Read the model definition and answer for the solid it produces. Units are mm, in the model's axes. Face numbers are marked on the shaded views. Coordinates: 2 decimals unless noted, no trailing zeros. Order: outer loops, then holes, each group sorted by start corner. A loop starts at its lowest first (then second) coordinate and runs counter-clockwise, first axis right, second up. Notation, with made-up numbers: (16, -32.5) -> (44, -32.5) arc R20 cw to (44, 0.5) -> close; hole circle Ø3 at (45.25, -31.75). An arc over 180 degrees is marked (long way). Use CSV: the item, a comma, the result in double quotes.
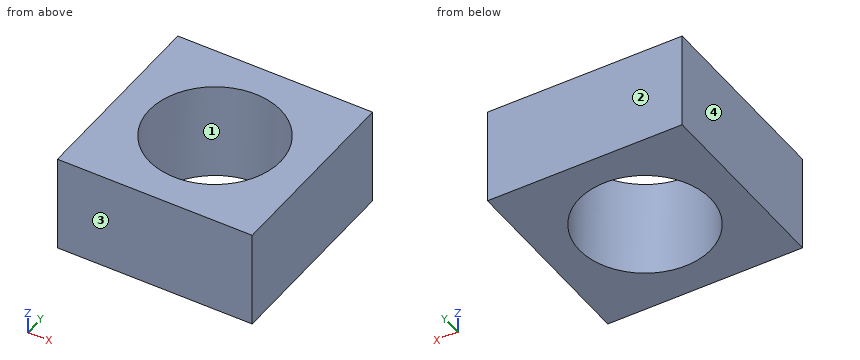
```python
from build123d import *

# Parameters (mm, degrees)
SKETCH2_W                       = 8
SKETCH2_H                       = 8
REFERENCE_SQUARE_NUT_DEPTH      = 4
SKETCH3_R                       = 2.7
SIMPLIFIED_CLEARANCE_BORE_DEPTH = 4


with BuildPart() as part:
    # Sketch2 → Reference_square_nut (new body)
    with BuildSketch(Plane.XY):
        Rectangle(SKETCH2_W, SKETCH2_H)
    extrude(amount=REFERENCE_SQUARE_NUT_DEPTH)

    # Sketch3 → Simplified_clearance_bore (cut)
    with BuildSketch(Plane.XY):
        Circle(SKETCH3_R)
    extrude(amount=SIMPLIFIED_CLEARANCE_BORE_DEPTH, mode=Mode.SUBTRACT)


solid = part.part
```
Item 1: Straight lines are drawn through the part: line 1 along Y through (x, z) = (0, 1.6); line 2 along X through (y, z) = (-0.5, 2.2); line 3 along Y through (x, z) = (-0.75, 3.6). For each, find the intervals that lie inside material, in ascending order.
Return value:
line 1,"y = -4 to -2.7, 2.7 to 4"
line 2,"x = -4 to -2.65, 2.65 to 4"
line 3,"y = -4 to -2.59, 2.59 to 4"
Item 2: The mould has two halves that part along Y. Classify the marked faces 1, 2, 3 and 4: +Y half, -Y half, draft (parallel to the pull), parting line (faces both ways), or undercut.
Return value:
face 1,"undercut"
face 2,"+Y half"
face 3,"-Y half"
face 4,"draft"
Item 3: Find section A-A, the plane x = 0. Give the vertices of the cut face in (y, z).
Return value:
outline,"(-4, 0) -> (-2.7, 0) -> (-2.7, 4) -> (-4, 4) -> close; (2.7, 0) -> (4, 0) -> (4, 4) -> (2.7, 4) -> close"
Item 4: Find section C-C, the plane z = 2.7. Give the vertices of the cut face in (x, y).
Return value:
outline,"(-4, -4) -> (4, -4) -> (4, 4) -> (-4, 4) -> close; hole circle Ø5.4 at (0, 0)"
